Can you work these out from the model? Positions are in its coordinate system, mm. Face numbers are marked on the shaded views. A direction names the side the tool comes from. Coordinates: 2 decimals unless noted, no trailing zeros. Order: outer loops, then holes, each group sorted by start corner. A loop starts at its lowest first (then second) coordinate and runs counter-clockwise, first axis right, second up. Notation, with made-up numbers: (-24, -1.75) - (-11, -1.75) arc R16 cw to (-11, 23.25) - close; hole circle Ø9 at (53.25, -1). An arc over 180 degrees is marked (long way). Return JSON: item names as keys, results as strings. Group by question number.
1) If we mould it in two halves opening along X, with no side actions, what happens to the marked faces 6, 7, 8 and 9? For each: pulls with the +X half, pulls with the -X half, needs draft (parallel to the pull), parting line crosses it, or undercut.
2) Imagine slicing it at B-B (x = 5.75). Write out the boundary of the cut face in (y, z).
3) Imagine slicing it at A-A (y = -15). Write out the boundary of the cut face in (x, z), and give its area (3 significant figures).
4) For pin 1 Ø0.6 at (x, z) = (5, 1) entering from -Y; pin 2 Ø1 at (x, z) = (2, 1) entering from -Y; pin 3 Ø0.6 at (y, z) = (1, 1) entering from +X; pin 4 Ø1 at (x, z) = (11.5, 1) entering from +Y, each with a flat end and sliding along its axis, tell me the tip position at first contact or that it passes through.
5) Which directions (+Z, -Z, +X, -X, +Y, -Y) give clear straight access to the entire face, cutting with the end or side of a thin tool? Please do the marked faces 1, 2, 3, 4 and 5.
6) Imagine slicing it at D-D (x = 9.75). Write out the boundary of the cut face in (y, z), and give its area (3 significant figures).
7) If I drill on line 1 along Y through (x, z) = (5.5, 0.65); line 2 along X through (y, z) = (-11.25, 1.55); line 3 along Y through (x, z) = (4.25, 1.6), over which ranges is the centre line in solid material (lowest first)?
8) Imagine slicing it at C-C (z = 1.2). Write out the boundary of the cut face in (x, y).
```python
from build123d import *

# Parameters (mm, degrees)
F0_W     = 2.236037234
F0_H     = 0.718915021
F1_DEPTH = 2


with BuildPart() as f1:
    # F0 (on Top) → F1 (new body)
    with BuildSketch(Plane.XY):
        Polygon((2.0192633942, 0.4625715956), (2.0192633942, -0.8831437444), (2.6445035461, -0.8831437444), (2.6445035461, -0.1642287234), (4.8805407801, -0.1642287234), (4.8805407801, -0.8831437444), (6.0192633942, -0.8831437444), (6.0192633942, 4.1168562556), (2.0192633942, 4.1168562556), (2.0192633942, 2.7711409156), (4.5192633942, 2.7711409156), (4.5192633942, 0.4625715956), align=None)
        Polygon((-1.9807366058, -0.8831437444), (2.0192633942, -0.8831437444), (2.0192633942, 0.4625715956), (-0.4807366058, 0.4625715956), (-0.4807366058, 2.7711409156), (2.0192633942, 2.7711409156), (2.0192633942, 4.1168562556), (-1.9807366058, 4.1168562556), align=None)
        with Locations((3.7625221631, -0.5236862339)):
            Rectangle(F0_W, F0_H)
        Polygon((4.8805407801, -0.8831437444), (2.6445035461, -0.8831437444), (2.6445035461, -19.4042553191), (4.8805407801, -19.4042553191), (4.8805407801, -10.3506205674), (15.0164007092, -10.3506205674), (15.0164007092, -19.4042553191), (17.2524379433, -19.4042553191), (17.2524379433, -0.1642287234), (15.0164007092, -0.1642287234), (15.0164007092, -8.3503989362), (4.8805407801, -8.3503989362), align=None)
    extrude(amount=F1_DEPTH)


solid = f1.part
```
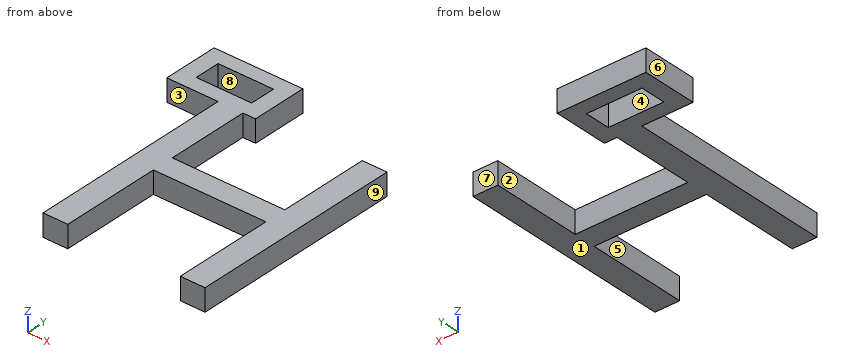
Calculated:
{
 "1": {"face 6": "pulls with the -X half", "face 7": "needs draft", "face 8": "undercut", "face 9": "pulls with the +X half"},
 "2": {"outline": "(-10.35, 0) - (-8.35, 0) - (-8.35, 2) - (-10.35, 2) - close; (-0.88, 0) - (4.12, 0) - (4.12, 2) - (-0.88, 2) - close"},
 "3": {"outline": "(2.64, 0) - (4.88, 0) - (4.88, 2) - (2.64, 2) - close; (15.02, 0) - (17.25, 0) - (17.25, 2) - (15.02, 2) - close", "area": "8.94 mm2"},
 "4": {"pin 1": "y = -19.4", "pin 2": "y = -0.88", "pin 3": "x = 6.02", "pin 4": "y = -8.35"},
 "5": {"face 1": "-Z, +X, -X, +Y, -Y", "face 2": "+Z, -Z, +Y", "face 3": "+Z, -Z, -X, -Y", "face 4": "+Z, -Z", "face 5": "+Z, -Z, -Y"},
 "6": {"outline": "(-10.35, 0) - (-8.35, 0) - (-8.35, 2) - (-10.35, 2) - close", "area": "4.00 mm2"},
 "7": {"line 1": "-10.35 to -8.35, -0.88 to 4.12", "line 2": "2.64 to 4.88, 15.02 to 17.25", "line 3": "-19.4 to 0.46, 2.77 to 4.12"},
 "8": {"outline": "(-1.98, -0.88) - (2.64, -0.88) - (2.64, -19.4) - (4.88, -19.4) - (4.88, -10.35) - (15.02, -10.35) - (15.02, -19.4) - (17.25, -19.4) - (17.25, -0.16) - (15.02, -0.16) - (15.02, -8.35) - (4.88, -8.35) - (4.88, -0.88) - (6.02, -0.88) - (6.02, 4.12) - (-1.98, 4.12) - close; hole (-0.48, 0.46) - (4.52, 0.46) - (4.52, 2.77) - (-0.48, 2.77) - close"}
}
